Work out the finished part from the listing and answer in its coordinate system (mm). A direction names the side the tool comes from. Coordinates: 2 decimals unless noted, no trailing zeros. Loops run counter-clockwise (first coordinate to the right, second up) from the corner with the lowest first, then second, coordinate; pieces in that order, holes last. Notation, with made-up numbers: M 89,33 L 101,33 A22 ccw 101,58 Z; hole C 82,44.25 d9. An arc over 180 degrees is marked long. Write each question's results on one line, items separated by ' | '.
```python
from build123d import *

# Parameters (mm, degrees)
F0_W     = 15
F0_H     = 5
F0_H_2   = 18
F1_DEPTH = 95


with BuildPart() as f1:
    # F0 (on Top) → F1 (new body)
    with BuildSketch(Plane.XY):
        Polygon((2, -18), (2, 18), (-2, 18), (-2, 14), (-2, 9), (-2, -9), (-2, -14), (-2, -18), align=None)
        with Locations((-9.5, 11.5)):
            Rectangle(F0_W, F0_H)
        with Locations((-9.5, 0)):
            Rectangle(F0_W, F0_H_2)
        with Locations((-9.5, -11.5)):
            Rectangle(F0_W, F0_H)
    extrude(amount=F1_DEPTH)


solid = f1.part
```
1) Find section C-C, the plane y = -15. Give the vertices of the cut face in (x, z).
Check result:
outline: M -2,0 L 2,0 L 2,95 L -2,95 Z
2) Straight lines are drawn through the part: probe 1 along Y at (x, z) = (-10.5, 88); probe 2 along X at (y, z) = (-15, 12.5). For each, find the intervals that lie inside material, in ascending order. Write a range as [from, to].
Check result:
probe 1: [-14, 14] | probe 2: [-2, 2]
3) Given pin 1 Ø5 at (x, z) = (-12, 59.5) entering from +Y; pin 2 Ø2 at (y, z) = (-17, 27) entering from -X; pin 3 Ø8 at (x, z) = (-7, 56) entering from -Y, each flat-ended and moving along its own axis, determine where each tip first touches the part or whether it passes through.
Check result:
pin 1: y = 14 | pin 2: x = -2 | pin 3: y = -14
4) Find section A-A, the plane z = 70. Give the vertices of the cut face in (x, y).
Check result:
outline: M -17,-14 L -2,-14 L -2,-18 L 2,-18 L 2,18 L -2,18 L -2,14 L -17,14 Z
5) Which of the six approach directions +Z, -Z, +X, -X, +Y, -Y give full straight-line access (tool end or side, diameter ignored) to faces 1 (the face through (-8, 0, 95)), 2 (the face through (-10, -14, 47)), 3 (the face through (-10, 14, 47))?
Check result:
face 1: +Z, +X, -X, +Y, -Y | face 2: +Z, -Z, -X, -Y | face 3: +Z, -Z, -X, +Y
6) Find section B-B, the plane x = -11.75. Give the vertices of the cut face in (y, z).
Check result:
outline: M -14,0 L 14,0 L 14,95 L -14,95 Z
